from build123d import *

# Parameters (mm, degrees)
F0_W        = 53.3761642873
F0_H        = 53.3400028944
F1_DEPTH    = 53.34
F4_T1_DEPTH = 591.1352105984


# Not quite as in the source:
# - a fillet or chamfer that OpenCascade refuses, or shapes differently, is made with other operations: its cross-section is extruded or revolved along the edge and cut away or added


with BuildPart() as f1:
    # F0 (on Front) → F1 (new body)
    with BuildSketch(Plane.XZ):
        with Locations((-26.6880821437, 26.6700014472)):
            Rectangle(F0_W, F0_H)
    extrude(amount=F1_DEPTH)

    # F2: F1 across plane


with BuildPart() as f1_1:
    add(f1.part)
    add(f1.part.mirror(Plane.YZ))

    # F3: F1 across face


with BuildPart() as f1_2:
    add(f1_1.part)
    add(f1_1.part.mirror(Plane(origin=(0, -53.34, 26.6700014472), x_dir=(1, 0, 0), z_dir=(0, -1, 0))))

    # F4: fillet of radius 114.6703157856 on 1 edges, made by hand

    # F4_s2 → F4_t1 (cut)
    with BuildSketch(Plane.XZ.offset(-242.2276052992)):
        with BuildLine():
            ThreePointArc((-43.5148778323, 53.3400028944), (11.7866365045, 39.1237753005), (53.3761642873, 0))
            Line((53.3761642873, 0), (53.3761642873, 53.3400028944))
            Line((53.3761642873, 53.3400028944), (-43.5148778323, 53.3400028944))
        make_face()
    extrude(amount=F4_T1_DEPTH, mode=Mode.SUBTRACT)


solid = f1_2.part
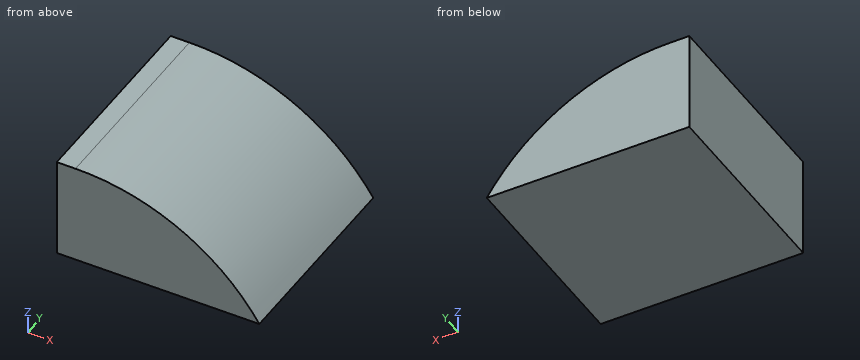
Input: part model. Units: mm. Frame: model coordinates. Coordinates: 2 decimals unless noted, no trailing zeros. Loops run counter-clockwise (first coordinate to the right, second up) from the corner with the lowest first, then second, coordinate; pieces in that order, holes last. Notation, with made-up numbers: (17.25, 84.5) -> (34.25, 84.5) arc R19 cw to (34.25, 109.5) -> close; hole circle Ø4 at (9, 0). An arc over 180 degrees is marked (long way). Write each question's results on one line, items separated by ' | '. Start each with the question number.
Q1. Ray query, line 1 (X direction, y = -70, z = 8.5); line 2 (Z direction, x = 6.5, y = -12); line 3 (Z direction, x = 29.5, y = -47.5). Return the intervals inside material, ascending. Write a range as from..to.
Q2. Section A-A, the plane y = -86. Return the cut outline in (x, z).
Q3. Section B-B, the plane x = 19.5. Return the cut outline in (y, z), plus the area to 3 significant figures.
Q4. Pin query (flat end, axial travel): pin 1 (3 mm diameter, centred on x = 38.5, y = -29.5, fed in from +Z). Return the tip coordinate at first contact, or that it passes through.
Found:
1) line 1: -53.38..47.44 | line 2: 0..41.86 | line 3: 0..27.09
2) outline: (-53.38, 0) -> (53.38, 0) arc R114.67 ccw to (-43.51, 53.34) -> (-53.38, 53.34) -> close
3) outline: (-106.68, 0) -> (0, 0) -> (0, 34.47) -> (-106.68, 34.47) -> close | area: 3,680 mm2
4) pin 1: z = 20.32
